For this review, use the dimensioned drawing (mm, ordinates from the lowest corner) and the shaded views. Coordinates: 2 decimals unless noted, no trailing zeros. Order: outer loops, then holes, each group sorted by start corner. A loop starts at its lowest first (then second) coordinate and runs counter-clockwise, first axis right, second up. Notation, with made-up numbers: M 52.25,-4.75 L 97.25,-4.75 A32 cw 97.25,33.25 Z; hole C 57.5,18.25 d10. An arc over 180 degrees is marked long. Use CSV: the item, a comma, the result in double quotes.
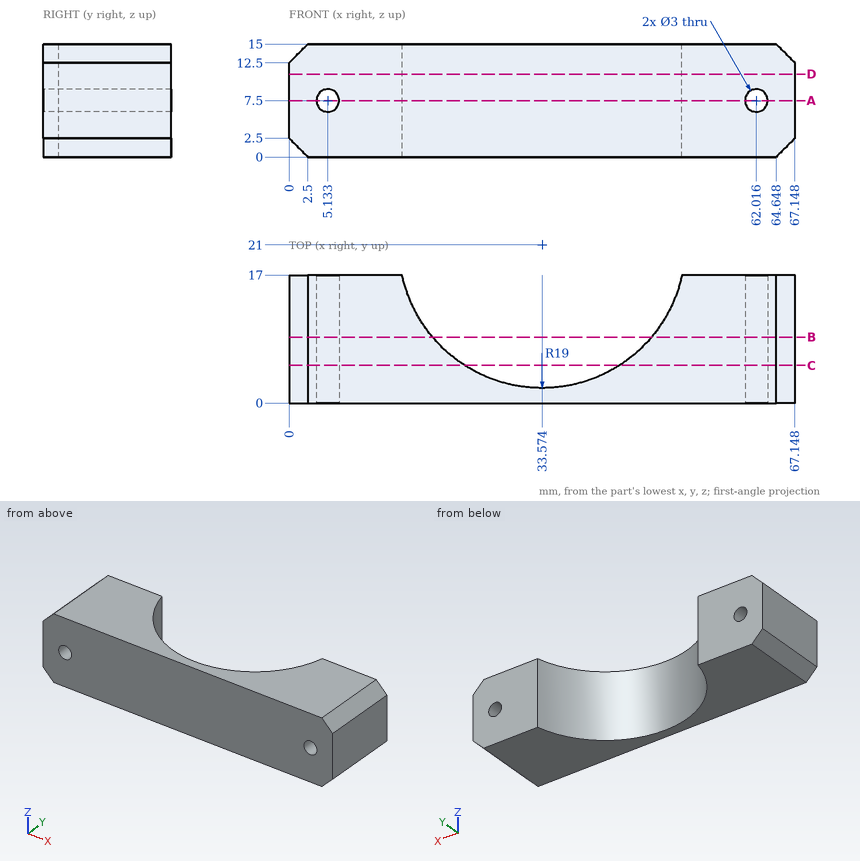
Item 1: Add section B-B on y = 8.75. State how many separate pieces and enclosed holes the cut face has, and give its area (3 significant figures).
Solutions:
separate pieces,"2"
enclosed holes,"2"
area,"545 mm^2"
Item 2: To check wall thickness, follow line 1 along Y through (x, z) = (34, 12.25) (1 decimal); line 2 along X through (y, z) = (15, 5.75) (1 decimal); line 3 along Z through (x, y) = (6, 8.5) (1 decimal). State the ranges of each line that lie inside material, in increasing order. Write a range as [from, to].
Solutions:
line 1,"[0, 2]"
line 2,"[0, 15.5], [51.6, 67.1]"
line 3,"[0, 6.3], [8.7, 15]"
Item 3: Clearance check with a flat-ended pin moving along its axis: pin 1 Ø10 at (x, y) = (23, 13) entering from +Z. State where the tip first meets the part, or that it passes through.
Solutions:
pin 1,"through"
Item 4: Add section A-A on z = 7.5. State the section outline as (x, y) points (1 decimal).
Solutions:
outline,"M 0,0 L 3.6,0 L 3.6,17 L 0,17 Z; M 6.6,0 L 60.5,0 L 60.5,17 L 52.1,17 A19 cw 15,17 L 6.6,17 Z; M 63.5,0 L 67.1,0 L 67.1,17 L 63.5,17 Z"
Item 5: Add section D-D on z = 11. State the section outline as (x, y) points (1 decimal).
Solutions:
outline,"M 0,0 L 67.1,0 L 67.1,17 L 52.1,17 A19 cw 15,17 L 0,17 Z"
Item 6: Add section C-C on y = 5. State the section outline as (x, z) points (1 decimal), and give its area (3 significant figures).
Solutions:
outline,"M 0,2.5 L 2.5,0 L 23.3,0 L 23.3,15 L 2.5,15 L 0,12.5 Z; M 43.8,0 L 64.6,0 L 67.1,2.5 L 67.1,12.5 L 64.6,15 L 43.8,15 Z; hole C 5.1,7.5 d3; hole C 62,7.5 d3"
area,"673 mm^2"
